from build123d import *

# Parameters (mm, degrees)
BOSS_EXTRUDE2_DEPTH = 2.5


with BuildPart() as part:
    # Sketch1 → Boss-Extrude2 (new body)
    with BuildSketch(Plane(origin=(0, 0, 0), x_dir=(1, 0, 0), z_dir=(0, 1, 0))):
        with BuildLine():
            ThreePointArc((-20.284442352, 5.435199947), (-14.849242405, 14.849242405), (-5.435199947, 20.284442352))
            Line((-5.435199947, 20.284442352), (-5.862251372, 21.878219965))
            ThreePointArc((-5.862251372, 21.878219965), (-16.015968594, 16.015968594), (-21.878219965, 5.862251372))
            Line((-21.878219965, 5.862251372), (-20.284442352, 5.435199947))
        make_face()
        with BuildLine():
            ThreePointArc((-20.284442352, -5.435199947), (-21, 0), (-20.284442352, 5.435199947))
            Line((-20.284442352, 5.435199947), (-21.878219965, 5.862251372))
            ThreePointArc((-21.878219965, 5.862251372), (-22.65, 0), (-21.878219965, -5.862251372))
            Line((-21.878219965, -5.862251372), (-20.284442352, -5.435199947))
        make_face()
        with BuildLine():
            Line((-5.862251372, -21.878219965), (-5.435199947, -20.284442352))
            ThreePointArc((-5.435199947, -20.284442352), (-14.849242405, -14.849242405), (-20.284442352, -5.435199947))
            Line((-20.284442352, -5.435199947), (-21.878219965, -5.862251372))
            ThreePointArc((-21.878219965, -5.862251372), (-16.015968594, -16.015968594), (-5.862251372, -21.878219965))
        make_face()
        with BuildLine():
            ThreePointArc((5.435199947, -20.284442352), (0, -21), (-5.435199947, -20.284442352))
            Line((-5.435199947, -20.284442352), (-5.862251372, -21.878219965))
            ThreePointArc((-5.862251372, -21.878219965), (0, -22.65), (5.862251372, -21.878219965))
            Line((5.862251372, -21.878219965), (5.435199947, -20.284442352))
        make_face()
        with BuildLine():
            Line((21.878219965, -5.862251372), (20.284442352, -5.435199947))
            ThreePointArc((20.284442352, -5.435199947), (14.849242405, -14.849242405), (5.435199947, -20.284442352))
            Line((5.435199947, -20.284442352), (5.862251372, -21.878219965))
            ThreePointArc((5.862251372, -21.878219965), (16.015968594, -16.015968594), (21.878219965, -5.862251372))
        make_face()
        with BuildLine():
            ThreePointArc((21, 0), (20.820342089, -2.741050037), (20.284442352, -5.435199947))
            Line((20.284442352, -5.435199947), (21.878219965, -5.862251372))
            ThreePointArc((21.878219965, -5.862251372), (22.45622611, -2.956418254), (22.65, 0))
            ThreePointArc((22.65, 0), (22.45622611, 2.956418254), (21.878219965, 5.862251372))
            Line((21.878219965, 5.862251372), (20.284442352, 5.435199947))
            ThreePointArc((20.284442352, 5.435199947), (20.820342089, 2.741050037), (21, 0))
        make_face()
        with BuildLine():
            Line((5.862251372, 21.878219965), (5.435199947, 20.284442352))
            ThreePointArc((5.435199947, 20.284442352), (14.849242405, 14.849242405), (20.284442352, 5.435199947))
            Line((20.284442352, 5.435199947), (21.878219965, 5.862251372))
            ThreePointArc((21.878219965, 5.862251372), (16.015968594, 16.015968594), (5.862251372, 21.878219965))
        make_face()
        with BuildLine():
            Line((0, 22.65), (0, 21))
            ThreePointArc((0, 21), (2.741050037, 20.820342089), (5.435199947, 20.284442352))
            Line((5.435199947, 20.284442352), (5.862251372, 21.878219965))
            ThreePointArc((5.862251372, 21.878219965), (2.956418254, 22.45622611), (0, 22.65))
        make_face()
        with BuildLine():
            ThreePointArc((-5.435199947, 20.284442352), (-2.741050037, 20.820342089), (0, 21))
            Line((0, 21), (0, 22.65))
            ThreePointArc((0, 22.65), (-2.956418254, 22.45622611), (-5.862251372, 21.878219965))
            Line((-5.862251372, 21.878219965), (-5.435199947, 20.284442352))
        make_face()
        with BuildLine():
            ThreePointArc((-11.446221042, 3.067005684), (-8.379215357, 8.379215357), (-3.067005684, 11.446221042))
            Line((-3.067005684, 11.446221042), (-4.141104722, 15.454813221))
            ThreePointArc((-4.141104722, 15.454813221), (-11.313708499, 11.313708499), (-15.454813221, 4.141104722))
            Line((-15.454813221, 4.141104722), (-11.446221042, 3.067005684))
        make_face()
        with BuildLine():
            ThreePointArc((-11.446221042, -3.067005684), (-11.85, 0), (-11.446221042, 3.067005684))
            Line((-11.446221042, 3.067005684), (-15.454813221, 4.141104722))
            ThreePointArc((-15.454813221, 4.141104722), (-16, 0), (-15.454813221, -4.141104722))
            Line((-15.454813221, -4.141104722), (-11.446221042, -3.067005684))
        make_face()
        with BuildLine():
            ThreePointArc((3.067005684, -11.446221042), (0, -11.85), (-3.067005684, -11.446221042))
            Line((-3.067005684, -11.446221042), (-4.141104722, -15.454813221))
            ThreePointArc((-4.141104722, -15.454813221), (0, -16), (4.141104722, -15.454813221))
            Line((4.141104722, -15.454813221), (3.067005684, -11.446221042))
        make_face()
        with BuildLine():
            Line((15.454813221, -4.141104722), (11.446221042, -3.067005684))
            ThreePointArc((11.446221042, -3.067005684), (8.379215357, -8.379215357), (3.067005684, -11.446221042))
            Line((3.067005684, -11.446221042), (4.141104722, -15.454813221))
            ThreePointArc((4.141104722, -15.454813221), (11.313708499, -11.313708499), (15.454813221, -4.141104722))
        make_face()
        with BuildLine():
            ThreePointArc((16, 0), (15.863117782, -2.088419076), (15.454813221, -4.141104722))
            Line((15.454813221, -4.141104722), (20.284442352, -5.435199947))
            ThreePointArc((20.284442352, -5.435199947), (20.820342089, -2.741050037), (21, 0))
            ThreePointArc((21, 0), (20.820342089, 2.741050037), (20.284442352, 5.435199947))
            Line((20.284442352, 5.435199947), (15.454813221, 4.141104722))
            ThreePointArc((15.454813221, 4.141104722), (15.863117782, 2.088419076), (16, 0))
        make_face()
        with BuildLine():
            ThreePointArc((11.85, 0), (11.748621607, -1.546735378), (11.446221042, -3.067005684))
            Line((11.446221042, -3.067005684), (15.454813221, -4.141104722))
            ThreePointArc((15.454813221, -4.141104722), (15.863117782, -2.088419076), (16, 0))
            ThreePointArc((16, 0), (15.863117782, 2.088419076), (15.454813221, 4.141104722))
            Line((15.454813221, 4.141104722), (11.446221042, 3.067005684))
            ThreePointArc((11.446221042, 3.067005684), (11.748621607, 1.546735378), (11.85, 0))
        make_face()
        with BuildLine():
            Line((0, 21), (0, 16))
            ThreePointArc((0, 16), (2.088419076, 15.863117782), (4.141104722, 15.454813221))
            Line((4.141104722, 15.454813221), (5.435199947, 20.284442352))
            ThreePointArc((5.435199947, 20.284442352), (2.741050037, 20.820342089), (0, 21))
        make_face()
        with BuildLine():
            ThreePointArc((-3.067005684, 11.446221042), (-1.546735378, 11.748621607), (0, 11.85))
            Line((0, 11.85), (0, 16))
            ThreePointArc((0, 16), (-2.088419076, 15.863117782), (-4.141104722, 15.454813221))
            Line((-4.141104722, 15.454813221), (-3.067005684, 11.446221042))
        make_face()
        with BuildLine():
            Line((0, 16), (0, 11.85))
            ThreePointArc((0, 11.85), (1.546735378, 11.748621607), (3.067005684, 11.446221042))
            Line((3.067005684, 11.446221042), (4.141104722, 15.454813221))
            ThreePointArc((4.141104722, 15.454813221), (2.088419076, 15.863117782), (0, 16))
        make_face()
        with BuildLine():
            Line((-4.141104722, -15.454813221), (-3.067005684, -11.446221042))
            ThreePointArc((-3.067005684, -11.446221042), (-8.379215357, -8.379215357), (-11.446221042, -3.067005684))
            Line((-11.446221042, -3.067005684), (-15.454813221, -4.141104722))
            ThreePointArc((-15.454813221, -4.141104722), (-11.313708499, -11.313708499), (-4.141104722, -15.454813221))
        make_face()
        with BuildLine():
            ThreePointArc((4.141104722, -15.454813221), (0, -16), (-4.141104722, -15.454813221))
            Line((-4.141104722, -15.454813221), (-5.435199947, -20.284442352))
            ThreePointArc((-5.435199947, -20.284442352), (0, -21), (5.435199947, -20.284442352))
            Line((5.435199947, -20.284442352), (4.141104722, -15.454813221))
        make_face()
        with BuildLine():
            ThreePointArc((-4.141104722, 15.454813221), (-2.088419076, 15.863117782), (0, 16))
            Line((0, 16), (0, 21))
            ThreePointArc((0, 21), (-2.741050037, 20.820342089), (-5.435199947, 20.284442352))
            Line((-5.435199947, 20.284442352), (-4.141104722, 15.454813221))
        make_face()
        with BuildLine():
            Line((4.141104722, 15.454813221), (3.067005684, 11.446221042))
            ThreePointArc((3.067005684, 11.446221042), (8.379215357, 8.379215357), (11.446221042, 3.067005684))
            Line((11.446221042, 3.067005684), (15.454813221, 4.141104722))
            ThreePointArc((15.454813221, 4.141104722), (11.313708499, 11.313708499), (4.141104722, 15.454813221))
        make_face()
        with BuildLine():
            ThreePointArc((-15.454813221, -4.141104722), (-16, 0), (-15.454813221, 4.141104722))
            Line((-15.454813221, 4.141104722), (-20.284442352, 5.435199947))
            ThreePointArc((-20.284442352, 5.435199947), (-21, 0), (-20.284442352, -5.435199947))
            Line((-20.284442352, -5.435199947), (-15.454813221, -4.141104722))
        make_face()
    extrude(amount=BOSS_EXTRUDE2_DEPTH)


solid = part.part
Could you check a few things on this model? Use its own coordinates, in mm. A direction names the side the tool comes from. Give positions to 0.01 mm unless a question says otherwise; leave off trailing zeros. Order: outer loops, then holes, each group sorted by start corner. A loop starts at its lowest first (then second) coordinate and runs counter-clockwise, first axis right, second up. Notation, with made-up numbers: (65, 78) -> (120, 78) arc R18 cw to (120, 106) -> close; hole circle Ø8 at (-3.5, 16). An arc over 180 degrees is marked (long way). Answer in a Markdown table with one row per item. Add a question column.
Item 1: Imagine slicing it at C-C (x = 16.5). List the corners of the cut face in (y, z) for me, and give its area (3 significant figures).
Item 2: For faces 1 (the flat face through (-7, 0, 10)), 2 (the flat face through (-17.84, 1.23, -4.78)), which set-ups out of +Z, -Z, +X, -X, +Y, -Y let a thin tool reach every point of the face, with its end or its side?
Item 3: Please list where these lines run through material, in increasing order: probe 1 along Z at (x, y) = (-7.5, 0.3); probe 2 along Z at (x, y) = (13, 1.9).
Item 4: I'm going to push a flat-ended pin straight in: P1, Ø1.5, axis at x = -17.5, y = 0.5, coming from the +Z side. Where does the tip first touch, or does it pass through?
Item 5: Imagine slicing it at A-A (x = 10). List the corners of the cut face in (y, z) for me, and give its area (3 significant figures).
Item 6: Imagine slicing it at B-B (z = -1). List the corners of the cut face in (x, y) for me, and give its area (3 significant figures).
Item 7: Imagine slicing it at D-D (y = 0.85). List the corners of the cut face in (x, z) for me.
Item 8: We'd pull the mould along X, two halves only. Please class faces 3 (the flat face through (-7, 2.5, 10)), 4 (the flat face through (17.84, 1.23, 4.78)): pulls with the +X half, pulls with the -X half, needs draft (parallel to the pull), parting line crosses it, or undercut.
Result:
| question | item | result |
|---|---|---|
| 1 | outline | (0, -15.52) -> (2.5, -15.52) -> (2.5, -12.99) -> (0, -12.99) -> close; (0, -4.42) -> (2.5, -4.42) -> (2.5, 4.42) -> (0, 4.42) -> close; (0, 12.99) -> (2.5, 12.99) -> (2.5, 15.52) -> (0, 15.52) -> close |
| 1 | area | 34.7 mm2 |
| 2 | face 1 | +Z, -Z, +X, -X, -Y |
| 2 | face 2 | +Y, -Y |
| 3 | probe 1 | -21.37 to -19.62, -14.13 to -9.17, 9.17 to 14.13, 19.62 to 21.37 |
| 3 | probe 2 | -18.55 to -16.49, -9.33 to 9.33, 16.49 to 18.55 |
| 4 | P1 | z = 15.25 |
| 5 | outline | (0, -20.32) -> (2.5, -20.32) -> (2.5, -18.47) -> (0, -18.47) -> close; (0, -12.49) -> (2.5, -12.49) -> (2.5, -6.36) -> (0, -6.36) -> close; (0, 6.36) -> (2.5, 6.36) -> (2.5, 12.49) -> (0, 12.49) -> close; (0, 18.47) -> (2.5, 18.47) -> (2.5, 20.32) -> (0, 20.32) -> close |
| 5 | area | 39.9 mm2 |
| 6 | outline | (-22.63, 0) -> (-11.81, 0) -> (-11.81, 2.5) -> (-22.63, 2.5) -> close; (11.81, 0) -> (22.63, 0) -> (22.63, 2.5) -> (11.81, 2.5) -> close |
| 6 | area | 54.1 mm2 |
| 7 | outline | circle Ø45.3 at (0, 0); hole (-20.28, -5.44) arc R21 ccw to (-5.44, -20.28) -> (-4.14, -15.45) arc R16 cw to (-15.45, -4.14) -> close; hole (-20.28, 5.44) -> (-15.45, 4.14) arc R16 cw to (-4.14, 15.45) -> (-5.44, 20.28) arc R21 ccw to start; hole circle Ø23.7 at (0, 0); hole (4.14, -15.45) -> (5.44, -20.28) arc R21 ccw to (20.28, -5.44) -> (15.45, -4.14) arc R16 cw to start; hole (4.14, 15.45) arc R16 cw to (15.45, 4.14) -> (20.28, 5.44) arc R21 ccw to (5.44, 20.28) -> close |
| 8 | face 3 | needs draft |
| 8 | face 4 | undercut |
